Autodesk Inventor part; units mm, degrees
ref_plane "YZ Plane" through (0, 0, 0) normal (1, 0, 0) x (0, 1, 0)
ref_plane "XZ Plane" through (0, 0, 0) normal (0, 1, 0) x (-1, 0, 0)
ref_plane "XY Plane" through (0, 0, 0) normal (0, 0, 1) x (1, 0, 0)
sketch "Sketch1" plane through (0, 0, 0) normal (0, 0, 1) x (1, 0, 0)
  point P0 (0, 0)
sketch "Sketch2" plane through (0, 0, 0) normal (0, 0, 1) x (1, 0, 0)
  line L0 (0, 0) -> (80, 0)
  line L1 (80, 0) -> (40, 250)
  line L2 (40, 250) -> (0, 0)
  dimension "d0" = 80
  dimension "d1" = 250
  dimension "d2" = 40
extrude "Extrusion1" add sketch "Sketch2" against normal blind 3
sketch "Sketch3" plane through (0, 0, -3) normal (0, 0, -1) x (-1, 0, 0)
  circle A0 centre (-40, 175) radius 7.5
  line L0 (-80, 0) -> (0, 0)
  point P0 (-40, 250)
  point P1 (-40, 0)
  dimension "d5" = 15
  dimension "d6" = 0
  dimension "d7" = 175
fillet "Fillet1" radius 10 1 edges at (40, 250, -1.5)
extrude "Extrusion2" add sketch "Sketch3" along normal blind 147
mirror "Mirror1" about plane through (40, 175, -150) normal (0, 0, -1) of "Extrusion2", "Extrusion1"
fillet "Fillet2" radius 10 1 edges at (40, 250, -298.5)
sketch "Sketch8" plane through (0, 0, 0) normal (0, 0, 1) x (1, 0, 0)
  line L0 (0, 0) -> (80, 0)
  line L1 (35, 0) -> (45, 0)
  line L2 (45, 0) -> (45, 10)
  line L3 (45, 10) -> (35, 10)
  line L4 (35, 10) -> (35, 0)
  point P0 (40, 0)
  point P1 (40, 10)
  point P2 (35, 5)
  dimension "d30" = 10
  dimension "d31" = 10
  dimension "d32" = 35
extrude "Extrusion7" add sketch "Sketch8" along normal blind 10
properties part number "stand"
Source: CAD feature listing. Evaluate the final solid. Frame: model axes, mm. A direction names the side the tool comes from. Coordinates: 2 decimals unless noted, no trailing zeros. Order: outer loops, then holes, each group sorted by start corner. A loop starts at its lowest first (then second) coordinate and runs counter-clockwise, first axis right, second up. Notation, with made-up numbers: M 40.25,69 L 99.25,69 A25 ccw 99.25,94 Z; hole C -33.5,-22.75 d2. An arc over 180 degrees is marked long. Write each question's results on one line, items separated by ' | '. Start each with the question number.
1. Section A-A, the plane x = 73. Return the cut outline in (y, z).
2. Draft query along Z for faces 1 (the face through (15.274, 95.46, -1.479)), 2 (the face through (40, 5, 10)), 3 (the face through (40.976, 167.564, -147.942)). Return one class per face: +Z half, -Z half, draft (parallel to the pull), parting line (faces both ways), or undercut.
3. Section D-D, the plane z = -192.5. Return the cut outline in (x, y), then the cut area to 3 significant figures.
4. Pin query (flat end, axial travel): pin 1 (24 mm diameter, centred on x = 29, y = 147.5, fed in from +Z); pin 2 (8 mm diameter, centred on x = 41.5, z = 5, fed in from +Y); pin 3 (11 mm diameter, centred on y = 6, z = 6.5, fed in from +X); pin 4 (8 mm diameter, centred on x = 53.5, z = -149.5, fed in from -Y). Return the tip coordinate at first contact, or that it passes through.
5. Section C-C, the plane x = 40. Return the cut outline in (y, z), then the cut area to 3 significant figures.
6. Reachability of faces 4 (the face through (40, 10, 5)), 5 (the face through (35, 5, 5)), 6 (the face through (45, 5, 5)), 7 (the face through (40, 0, 0)) from +Z, -Z, +X, -X, +Y, -Y: full face, straight path, thin tool, end or side. Return the list, or none.
7. Material intervals for L1, parallel to Z at x = 41, y = 76; L2, parallel to Z at x = 38, y = 182; L3, parallel to Y at x = 46.5, z = -32, sorted ascending.
8. Section B-B, the plane y = 164. Return the cut outline in (x, z), then the cut area to 3 significant figures.
Solution:
1) outline: M 0,-300 L 43.75,-300 L 43.75,-297 L 0,-297 Z; M 0,-3 L 43.75,-3 L 43.75,0 L 0,0 Z
2) face 1: draft | face 2: +Z half | face 3: undercut
3) outline: C 40,175 d15 | area: 177 mm²
4) pin 1: z = 0 | pin 2: y = 10 | pin 3: x = 45 | pin 4: through
5) outline: M 0,-300 L 196.71,-300 L 196.71,-297 L 182.5,-297 L 182.5,-3 L 196.71,-3 L 196.71,0 L 10,0 L 10,10 L 0,10 L 0,-3 L 167.5,-3 L 167.5,-297 L 0,-297 Z | area: 5,690 mm²
6) face 4: +Z, +X, -X, +Y | face 5: +Z, -X, +Y, -Y | face 6: +Z, +X, +Y, -Y | face 7: +Z, -Z, +X, -X, -Y
7) L1: -300 to -297, -3 to 0 | L2: -300 to 0 | L3: 171.26 to 178.74
8) outline: M 26.24,-300 L 53.76,-300 L 53.76,-297 L 26.24,-297 Z; M 26.24,-3 L 53.76,-3 L 53.76,0 L 26.24,0 Z | area: 165 mm²
